Build history of the part. All positions in model axes, mm. A direction names the side the tool comes from. Round coordinates to 2 decimals unless told otherwise and drop trailing zeros. Write each loop counter-clockwise with the first axis right and the second up, starting at its lowest first coordinate (ties: lowest second). Pieces come first, ordered by that corner, then holes. Notation, with made-up numbers: (63, -6) -> (101, -6) arc R33 cw to (101, 27) -> close; hole circle Ø11 at (-7.75, -30.5). An arc over 180 degrees is marked (long way). Answer in a Markdown table with one row per item.
```python
from build123d import *

# Parameters (mm, degrees)
BOSS_EXTRUDE2_DEPTH = 30
FILLET1_R           = 3


with BuildPart() as part:
    # Sketch1 → Boss-Extrude2 (new body)
    with BuildSketch(Plane(origin=(0, 0, 0), x_dir=(0, 0, -1), z_dir=(1, 0, 0))):
        Polygon((0, 8), (0, 38), (8, 38), (8, 8), (38, 8), (38, 38), (46, 38), (46, 8), (61, 8), (61, 0), (-15, 0), (-15, 8), align=None)
    extrude(amount=BOSS_EXTRUDE2_DEPTH)

    # Fillet1
    fillet1_edges = [part.edges().sort_by_distance(p)[0] for p in [
        (15, 8, 15),
        (15, 8, 0),
        (15, 38, 0),
        (15, 38, -8),
        (15, 38, -38),
        (15, 38, -46),
        (15, 8, -46),
        (15, 8, -61),
    ]]
    fillet(fillet1_edges, radius=FILLET1_R)


solid = part.part
```
Q1. Saw through at A-A on y = 25. Write the cut outline in (x, z), plus the area to 3 significant figures.
A:
| item | result |
|---|---|
| outline | (0, -46) -> (30, -46) -> (30, -38) -> (0, -38) -> close; (0, -8) -> (30, -8) -> (30, 0) -> (0, 0) -> close |
| area | 480 mm² |
Q2. Drop flat-ended pins along their axis: P1, Ø10, axis at x = 14.5, z = -54.5, coming from the +Y side; P2, Ø8, axis at x = 22, y = 17, coming from the -Z side; P3, Ø13.5, axis at x = 15, y = 25, coming from the +Z side; P4, Ø1, axis at y = 11.5, z = -45.5, coming from the -X side. Give the stop position or say it passes through.
A:
| item | result |
|---|---|
| P1 | y = 8 |
| P2 | z = -46 |
| P3 | z = 0 |
| P4 | x = 0 |
Q3. Saw through at C-C on z = -50. Write the cut outline in (x, y).
A:
| item | result |
|---|---|
| outline | (0, 0) -> (30, 0) -> (30, 8) -> (0, 8) -> close |
Q4. Wall check: line 1 (Z direction, x = 7.25, y = 33.5); line 2 (Y direction, x = 19.75, z = -21); line 3 (Z direction, x = 8.5, y = 10). Give the ranges that are in metal, low to high. Write a range as [from, to].
A:
| item | result |
|---|---|
| line 1 | [-46, -38], [-8, 0] |
| line 2 | [0, 8] |
| line 3 | [-46.17, -38], [-8, 0.17] |
Q5. Which spindle directions (+Z, -Z, +X, -X, +Y, -Y) get a long thin tool onto all of the face, cutting with end or side? Do faces 1 (the flat face through (15, 8, 8)), 2 (the flat face through (0, 7, -24)), 3 (the flat face through (15, 8, -53)), 4 (the flat face through (30, 7, -24)), 5 (the cylindrical face through (15.21, 37.14, -7.1)). Say none if no direction does.
A:
| item | result |
|---|---|
| face 1 | +Z, +X, -X, +Y |
| face 2 | +Z, -Z, -X, +Y, -Y |
| face 3 | -Z, +X, -X, +Y |
| face 4 | +Z, -Z, +X, +Y, -Y |
| face 5 | +X, -X, +Y |
Q6. Saw through at D-D on y = 7. Write the cut outline in (x, z), plus the area to 3 significant figures.
A:
| item | result |
|---|---|
| outline | (0, -60.24) -> (30, -60.24) -> (30, 14.24) -> (0, 14.24) -> close |
| area | 2,230 mm² |
Q7. Saw through at B-B on x = 4. Write the cut outline in (y, z).
A:
| item | result |
|---|---|
| outline | (0, -61) -> (5, -61) arc R3 ccw to (8, -58) -> (8, -49) arc R3 cw to (11, -46) -> (35, -46) arc R3 ccw to (38, -43) -> (38, -41) arc R3 ccw to (35, -38) -> (8, -38) -> (8, -8) -> (35, -8) arc R3 ccw to (38, -5) -> (38, -3) arc R3 ccw to (35, 0) -> (11, 0) arc R3 cw to (8, 3) -> (8, 12) arc R3 ccw to (5, 15) -> (0, 15) -> close |
Q8. Two-plate mould, pull along Z, no slides. Class faces 6 (the cylindrical face through (15.21, 7.1, 14.14)), 7 (the flat face through (15, 21, -38)), 8 (the flat face through (15, 38, -4)): released by +Z, released by -Z, zero draft, split by the parting line, or undercut.
A:
| item | result |
|---|---|
| face 6 | released by +Z |
| face 7 | undercut |
| face 8 | zero draft |
